Here's the drawing with two shaded views (mm, measured from the low corner). I have some questions. A direction names the side the tool comes from. Coordinates: 2 decimals unless noted, no trailing zeros. Write each loop counter-clockwise with the first axis right and the second up, starting at its lowest first coordinate (ties: lowest second). Pieces come first, ordered by that corner, then holes.
Item 1: I'm going to push flat-ended pins straight in: pin 1 Ø4 at (x, z) = (15, 25) entering from +Y; pin 2 Ø5 at (y, z) = (7.5, 5) entering from +X; pin 3 Ø1.5 at (x, y) = (7, 1.5) entering from +Z; pin 4 Ø2.5 at (x, y) = (17.5, 6) entering from -Z. Where does each tip first touch, or does it pass through?
Item 2: If we section it at C-C (x = 14.5): Please give me the cut outline in (y, z), then the cut area to 3 significant figures.
Item 3: We'd pull the mould along X, two halves only. Please class the marked faces 1, 2, 3 and 4: +X half, -X half, draft (parallel to the pull), parting line (faces both ways), or undercut.
Item 4: If we section it at A-A (z = 24): Please give me the cut outline in (x, y).
Item 5: If I drill on line 1 (X direction, y = 7.75, z = 25); line 2 (X direction, y = 2.5, z = 12); line 3 (Z direction, x = 14.5, y = 8), over which ranges is the centre line in solid material (lowest first)?
Item 6: If we section it at D-D (z = 3.25): Please give me the cut outline in (x, y), then the cut area to 3 significant figures.
Item 7: If we section it at B-B (y = 1.5): Please give me the cut outline in (x, z), then the cut area to 3 significant figures.
Item 8: For the marked faces 5 and 6, which set-ups out of +Z, -Z, +X, -X, +Y, -Y let a thin tool reach every point of the face, with its end or its side?
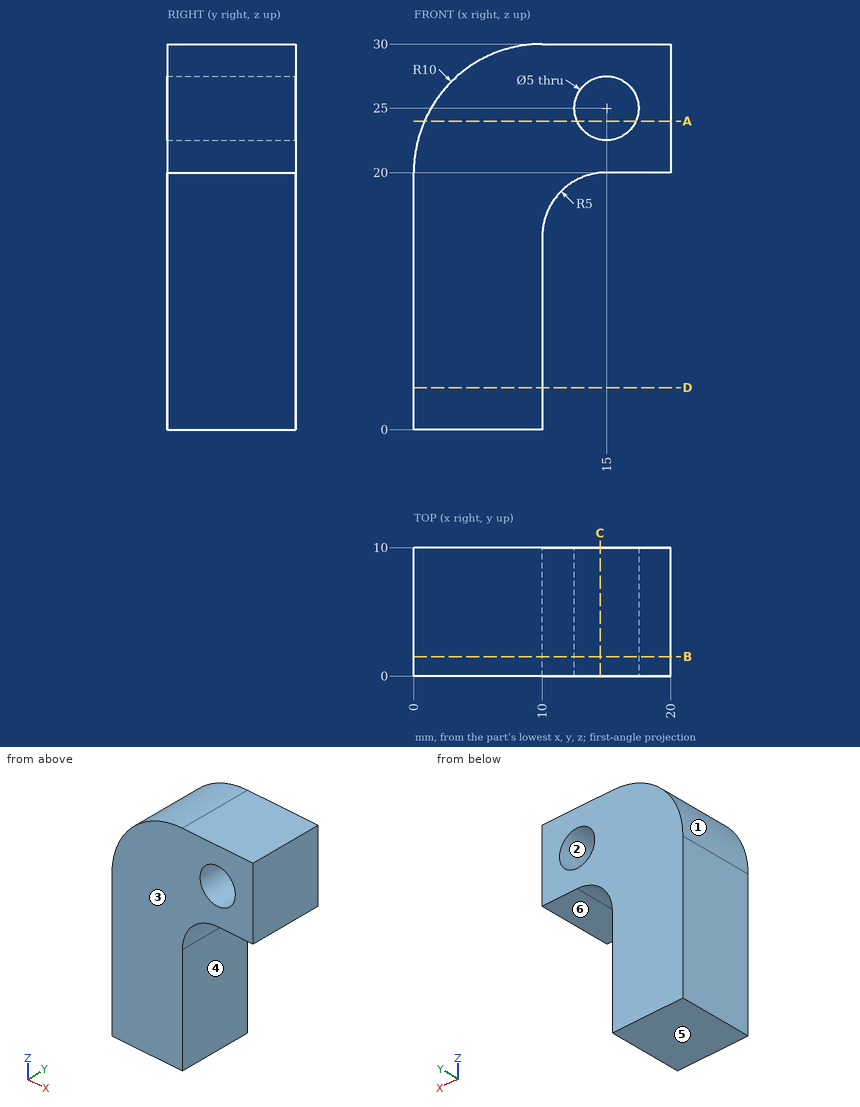
Answer list:
1. pin 1: passes through
1. pin 2: stops at x = 10
1. pin 3: stops at z = 29.74
1. pin 4: stops at z = 20
2. outline: (0, 19.97) - (10, 19.97) - (10, 22.55) - (0, 22.55) - close; (0, 27.45) - (10, 27.45) - (10, 30) - (0, 30) - close
2. area: 51.3 mm2
3. face 1: -X half
3. face 2: undercut
3. face 3: draft
3. face 4: +X half
4. outline: (0.83, 0) - (12.71, 0) - (12.71, 10) - (0.83, 10) - close; (17.29, 0) - (20, 0) - (20, 10) - (17.29, 10) - close
5. line 1: x = 1.34 to 12.5, 17.5 to 20
5. line 2: x = 0 to 10
5. line 3: z = 19.97 to 22.55, 27.45 to 30
6. outline: (0, 0) - (10, 0) - (10, 10) - (0, 10) - close
6. area: 100 mm2
7. outline: (0, 0) - (10, 0) - (10, 15) arc R5 cw to (15, 20) - (20, 20) - (20, 30) - (10, 30) arc R10 ccw to (0, 20) - close; hole circle Ø5 at (15, 25)
7. area: 364 mm2
8. face 5: -Z, +X, -X, +Y, -Y
8. face 6: -Z, +X, +Y, -Y
